```python
from build123d import *

# Parameters (mm, degrees)
BOSS_EXTRUDE1_DEPTH = 25.4
SKETCH2_R           = 1
CUT_EXTRUDE1_DEPTH  = 25.4
SKETCH2_4_R         = 1
CUT_EXTRUDE2_DEPTH  = 25.4
SKETCH2_5_R         = 1
CUT_EXTRUDE3_DEPTH  = 25.4
SKETCH2_6_R         = 1
CUT_EXTRUDE4_DEPTH  = 25.4
SKETCH3_R           = 1
CUT_EXTRUDE5_DEPTH  = 25.4


with BuildPart() as part:
    # Sketch1 → Boss-Extrude1 (new body)
    with BuildSketch(Plane(origin=(0, 0, 0), x_dir=(1, 0, 0), z_dir=(0, 1, 0))):
        Polygon((0, 0), (0, -2.54), (25.4, -2.54), (25.4, 0), (2.703011542, 0), (2.386819257, 0.868731164), (-6.858024694, 26.268731164), (-9.24484395, 25.4), align=None)
    extrude(amount=BOSS_EXTRUDE1_DEPTH)

    # Sketch2 → Cut-Extrude1 (cut)
    with BuildSketch(Plane(origin=(0, 0, 0), x_dir=(0.3420201433256697, 0, 0.9396926207859081), z_dir=(-0.939692620785908, 0, 0.34202014332566966))):
        with Locations((-17.604115421, 2)):
            Circle(SKETCH2_R)
    extrude(amount=-CUT_EXTRUDE1_DEPTH, mode=Mode.SUBTRACT)

    # Sketch2_4 → Cut-Extrude2 (cut)
    with BuildSketch(Plane(origin=(0, 0, 0), x_dir=(0.3420201433256697, 0, 0.9396926207859081), z_dir=(-0.939692620785908, 0, 0.34202014332566966))):
        with Locations((-17.604115421, 23.4)):
            Circle(SKETCH2_4_R)
    extrude(amount=-CUT_EXTRUDE2_DEPTH, mode=Mode.SUBTRACT)

    # Sketch2_5 → Cut-Extrude3 (cut)
    with BuildSketch(Plane(origin=(0, 0, 0), x_dir=(0.3420201433256697, 0, 0.9396926207859081), z_dir=(-0.939692620785908, 0, 0.34202014332566966))):
        with Locations((-3.104115421, 2)):
            Circle(SKETCH2_5_R)
    extrude(amount=-CUT_EXTRUDE3_DEPTH, mode=Mode.SUBTRACT)

    # Sketch2_6 → Cut-Extrude4 (cut)
    with BuildSketch(Plane(origin=(0, 0, 0), x_dir=(0.3420201433256697, 0, 0.9396926207859081), z_dir=(-0.939692620785908, 0, 0.34202014332566966))):
        with Locations((-3.104115421, 23.4)):
            Circle(SKETCH2_6_R)
    extrude(amount=-CUT_EXTRUDE4_DEPTH, mode=Mode.SUBTRACT)

    # Sketch3 → Cut-Extrude5 (cut)
    with BuildSketch(Plane(origin=(0, 0, 0), x_dir=(-1, 0, 0), z_dir=(0, 0, -1))):
        with Locations((-21.001496496, 21.59)):
            Circle(SKETCH3_R)
        with Locations((-21.001496496, 3.81)):
            Circle(SKETCH3_R)
        with Locations((-8.301496496, 21.59)):
            Circle(SKETCH3_R)
        with Locations((-8.301496496, 3.81)):
            Circle(SKETCH3_R)
    extrude(amount=-CUT_EXTRUDE5_DEPTH, mode=Mode.SUBTRACT)


solid = part.part
```
Design review of the part built by this model. Coordinates are the model's own, in mm. A direction names the side the tool comes from. Give positions to 0.01 mm unless a question says otherwise; leave off trailing zeros. Order: outer loops, then holes, each group sorted by start corner. A loop starts at its lowest first (then second) coordinate and runs counter-clockwise, first axis right, second up. Notation, with made-up numbers: (-4.5, 19) -> (47.5, 19) arc R11 cw to (47.5, 40) -> close; hole circle Ø2 at (16.5, -7). An arc over 180 degrees is marked (long way). Write item = value, one per line. Start each with the question number.
(1) For pin 1 (1.5 mm diameter, centred on y = 9.5, z = -1.5, fed in from +X); pin 2 (1 mm diameter, centred on x = 14.5, y = 7.5, fed in from -Z); pin 3 (1.2 mm diameter, centred on x = 21, y = 21.59, fed in from -Z); pin 4 (12 mm diameter, centred on y = 22.5, z = -4.5, fed in from -X), all flat-tipped, find the tip position at first contact; note any pin that passes through.
(2) To check wall thickness, follow line 1 along Z through (x, y) = (23, 11); line 2 along X through (y, z) = (10.5, 0.5); line 3 along X through (y, z) = (22.25, -4.75). State the ranges of each line that lie inside material, in increasing order.
(3) Mouldability with a two-part tool opening along Y and no side actions: class faces 1 (the face through (0, 25.4, -6)), 2 (the face through (-5.116, 1.392, -17.716)), 3 (the face through (0, 0, -6)), 4 (the face through (9.3, 3.85, 1.25)) as +Y half, -Y half, draft (parallel to the pull), parting line (faces both ways), or undercut.
(4) We need section B-B on x = 14. Write out the cut boundary in (y, z).
(5) We need section C-C on z = -3.5. State how many separate pieces and enclosed holes the cut face has, plus the area to 3 significant figures.
(6) For faces 5 (the face through (0, 13, 1)), 6 (the face through (-4.89, 24.39, -17.09)), 7 (the face through (14, 13, 0)), list the 3-axis set-ups (+Z, -Z, +X, -X, +Y, -Y) from which the entire face can be reached by the end or side of a thin tool; tool diameter is ignored.
(7) We need section A-A on y = 21.59. Write out the cut boundary in (x, z).
Numbers:
q1.pin_1 = 2.43
q1.pin_2 = 0
q1.pin_3 = through
q1.pin_4 = -3.82
q2.line_1 = 0 to 2.54
q2.line_2 = 0 to 25.4
q2.line_3 = -1.73 to 0.97
q3.face_1 = +Y half
q3.face_2 = undercut
q3.face_3 = -Y half
q3.face_4 = undercut
q4.outline = (0, 0) -> (25.4, 0) -> (25.4, 2.54) -> (0, 2.54) -> close
q5.separate_pieces = 3
q5.enclosed_holes = 0
q5.area = 58.4 mm^2
q6.face_5 = +Z, -X, +Y, -Y
q6.face_6 = none
q6.face_7 = -Z, +X, +Y, -Y
q7.outline = (-9.24, -25.4) -> (-6.86, -26.27) -> (2.7, 0) -> (7.3, 0) -> (7.3, 2.54) -> (0, 2.54) -> (0, 0) -> close; (9.3, 0) -> (20, 0) -> (20, 2.54) -> (9.3, 2.54) -> close; (22, 0) -> (25.4, 0) -> (25.4, 2.54) -> (22, 2.54) -> close
